Could you check a few things on this model? Use its own coordinates, in mm. Round coordinates to 2 decimals unless told otherwise and drop trailing zeros. Loops run counter-clockwise (first coordinate to the right, second up) from the corner with the lowest first, then second, coordinate; pieces in that order, holes last. Notation, with made-up numbers: (88, 61.5) - (110, 61.5) arc R24 cw to (110, 85.5) - close; hole circle Ø7 at (60.25, -34.5). An arc over 180 degrees is marked (long way). Answer as CSV lines item,"result". Start each with the question number.
1) We'd pull the mould along Y, two halves only. Please class faces 1 (the face through (-24.93, -112.265, 4.93)), 2 (the face through (-91.554, -30.723, 4.93)): pulls with the +Y half, pulls with the -Y half, needs draft (parallel to the pull), parting line crosses it, or undercut.
2) I'm going to push flat-ended pins straight in: pin 1 Ø2 at (y, z) = (19, 1.5) entering from +X; pin 2 Ø4 at (x, z) = (-73.5, 7) entering from +Y; pin 3 Ø4 at (x, z) = (54.5, 6.5) entering from +Y. Where does each tip first touch, or does it pass through?
3) Suppose I cut it at B-B, the plane x = 3. Write out the boundary of the cut face in (y, z).
4) Suppose I cut it at D-D, the plane z = 8.5. Count the separate pieces of the cut face and the enclosed holes in it, then the cut area to 3 significant figures.
5) Suppose I cut it at C-C, the plane y = -16. Write out the boundary of the cut face in (x, z), then the cut area to 3 significant figures.
6) Please list where these lines run through material, in increasing order: line 1 along Y through (x, z) = (0, 5.25); line 2 along Y through (x, z) = (-14.5, 9); line 3 along X through (y, z) = (-15.5, 4.5).
7) Suppose I cut it at A-A, the plane y = -83. Write out the boundary of the cut face in (x, z).
```python
from build123d import *

# Parameters (mm, degrees)
SKETCH1_R           = 115
BOSS_EXTRUDE1_DEPTH = 10
SKETCH3_R           = 6.25
SKETCH3_R_2         = 6.5
SKETCH3_R_3         = 42
CUT_EXTRUDE2_DEPTH  = 163.941707368


with BuildPart() as part:
    # Sketch1 → Boss-Extrude1 (new body)
    with BuildSketch(Plane.XY):
        Circle(SKETCH1_R)
    extrude(amount=BOSS_EXTRUDE1_DEPTH)

    # Sketch3 → Cut-Extrude2 (cut, through all)
    with BuildSketch(Plane.XY):
        with BuildLine():
            Line((18.484325558, 85.403687954), (22.603174126, 50.140767041))
            ThreePointArc((22.603174126, 50.140767041), (32.574916184, 44.315627442), (41.110477128, 36.536675688))
            Line((41.110477128, 36.536675688), (75.793703221, 44.120364278))
            ThreePointArc((75.793703221, 44.120364278), (79.175021421, 49.09862209), (78.573775649, 55.086515471))
            ThreePointArc((78.573775649, 55.086515471), (55.629022762, 78.938176107), (25.371814654, 92.349542839))
            ThreePointArc((25.371814654, 92.349542839), (20.87622799, 89.919618918), (18.484325558, 85.403687954))
        make_face()
        with BuildLine():
            ThreePointArc((-40.701938294, 36.991245168), (-32.080463562, 44.674868301), (-22.044607418, 50.388840866))
            Line((-22.044607418, 50.388840866), (-18.539417586, 85.718037702))
            ThreePointArc((-18.539417586, 85.718037702), (-22.229137331, 90.472228676), (-28.109757511, 91.750770782))
            ThreePointArc((-28.109757511, 91.750770782), (-57.884353357, 77.299582515), (-79.989312588, 52.667607817))
            ThreePointArc((-79.989312588, 52.667607817), (-79.067530287, 47.641163039), (-75.511763217, 43.970829232))
            Line((-75.511763217, 43.970829232), (-40.701938294, 36.991245168))
        make_face()
        with BuildLine():
            ThreePointArc((-47.7583554, -27.278920241), (-52.40173304, -16.70504039), (-54.73479378, -5.394659379))
            Line((-54.73479378, -5.394659379), (-87.251693421, 8.856296471))
            ThreePointArc((-87.251693421, 8.856296471), (-92.913383832, 6.81629027), (-95.946561206, 1.618579367))
            ThreePointArc((-95.946561206, 1.618579367), (-91.403520553, -31.164406796), (-74.80792857, -59.799171102))
            ThreePointArc((-74.80792857, -59.799171102), (-69.742649114, -60.475760896), (-65.153161777, -58.228220975))
            Line((-65.153161777, -58.228220975), (-47.7583554, -27.278920241))
        make_face()
        with BuildLine():
            ThreePointArc((11.18565141, -53.850545053), (-0.305588527, -54.999151045), (-11.783355506, -53.72292372))
            Line((-11.783355506, -53.72292372), (-35.385094524, -80.244545469))
            ThreePointArc((-35.385094524, -80.244545469), (-35.194491887, -86.259529612), (-31.188478418, -90.75043372))
            ThreePointArc((-31.188478418, -90.75043372), (1.393870963, -96.560245154), (33.755470104, -89.625528057))
            ThreePointArc((33.755470104, -89.625528057), (35.964202669, -85.017238768), (35.244894765, -79.957848899))
            Line((35.244894765, -79.957848899), (11.18565141, -53.850545053))
        make_face()
        with BuildLine():
            Line((86.935704672, 8.811552688), (54.671468158, -6.002546915))
            ThreePointArc((54.671468158, -6.002546915), (52.212868944, -17.286304309), (47.452279576, -27.807933455))
            Line((47.452279576, -27.807933455), (65.38250231, -58.450152982))
            ThreePointArc((65.38250231, -58.450152982), (71.161991629, -60.127611424), (76.671021486, -57.7054319))
            ThreePointArc((76.671021486, -57.7054319), (92.264980185, -28.513106671), (95.6699564, 4.407548503))
            ThreePointArc((95.6699564, 4.407548503), (91.969748742, 7.932217708), (86.935704672, 8.811552688))
        make_face()
        with Locations((52.308108396, 16.995934691)):
            Circle(SKETCH3_R)
        with Locations((0, 55)):
            Circle(SKETCH3_R_2)
        with Locations((-52.308108396, 16.995934691)):
            Circle(SKETCH3_R)
        with Locations((-32.328188876, -44.495934691)):
            Circle(SKETCH3_R)
        with Locations((32.328188876, -44.495934691)):
            Circle(SKETCH3_R)
        Circle(SKETCH3_R_3)
    extrude(amount=CUT_EXTRUDE2_DEPTH, mode=Mode.SUBTRACT)


solid = part.part
```
Filled sheet:
1,face 1,"parting line crosses it"
1,face 2,"undercut"
2,pin 1,"x = 113.58"
2,pin 2,"y = 90.07"
2,pin 3,"y = 102.32"
3,outline,"(-114.96, 0) - (-96.52, 0) - (-96.52, 10) - (-114.96, 10) - close; (-54.92, 0) - (-41.89, 0) - (-41.89, 10) - (-54.92, 10) - close; (41.89, 0) - (49.23, 0) - (49.23, 10) - (41.89, 10) - close; (60.77, 0) - (114.96, 0) - (114.96, 10) - (60.77, 10) - close"
4,separate pieces,"1"
4,enclosed holes,"11"
4,area,"24,400 mm²"
5,outline,"(-113.88, 0) - (-95.12, 0) - (-95.12, 10) - (-113.88, 10) - close; (-52.62, 0) - (-38.83, 0) - (-38.83, 10) - (-52.62, 10) - close; (38.83, 0) - (52.62, 0) - (52.62, 10) - (38.83, 10) - close; (95.09, 0) - (113.88, 0) - (113.88, 10) - (95.09, 10) - close"
5,area,"651 mm²"
6,line 1,"-115 to -96.57, -55 to -42, 42 to 48.5, 61.5 to 115"
6,line 2,"-114.08 to -95.36, -56.78 to -39.42, 39.42 to 114.08"
6,line 3,"-113.95 to -95.2, -52.77 to -39.04, 39.04 to 52.77, 95.16 to 113.95"
7,outline,"(-79.6, 0) - (-35.82, 0) - (-35.82, 10) - (-79.6, 10) - close; (36.04, 0) - (79.6, 0) - (79.6, 10) - (36.04, 10) - close"
